Autodesk Inventor part; units mm, degrees
ref_plane "YZ Plane" through (0, 0, 0) normal (1, 0, 0) x (0, 1, 0)
ref_plane "XZ Plane" through (0, 0, 0) normal (0, 1, 0) x (-1, 0, 0)
ref_plane "XY Plane" through (0, 0, 0) normal (0, 0, 1) x (1, 0, 0)
sketch "Sketch1" plane through (0, 0, 0) normal (1, 0, 0) x (0, 1, 0)
  line L0 (10, 0) -> (10, -13)
  line L1 (0, 0) -> (0, -13)
  line L2 (52, -13) -> (52, 55)
  line L3 (52, 55) -> (32, 55)
  line L4 (52, 55) -> (72, 55) construction
  line L5 (32, 55) -> (32, 40)
  line L6 (32, 55) -> (47, 55) construction
  line L7 (32, 40) -> (32, 40)
  line L8 (42, 30) -> (42, -13)
  arc A0 (42, 30) -> (32, 40) centre (32, 30) ccw
  arc A1 (10, -13) -> (42, -13) centre (26, -13) ccw
  arc A2 (0, -13) -> (52, -13) centre (26, -13) ccw
  line L9 (0, 0) -> (10, 0)
  dimension "d2" = 13
  dimension "d7" = 13
  dimension "d12" = 68
  dimension "d14" = 20
  dimension "d16" = 15
  dimension "d19" = 10
  dimension "d20" = 16
  dimension "d21" = 26
  dimension "d22" = 10
extrude "Extrusion1" add sketch "Sketch1" along normal blind 50
sketch "Sketch2" plane through (0, 32, 40) normal (0, -1, 0) x (1, 0, 0)
  circle A0 centre (10, 7.5) radius 2
  line L0 (0, 15) -> (0, 0)
  line L1 (0, 15) -> (50, 15)
  circle A1 centre (40, 7.5) radius 2
  point P0 (0, -40)
  dimension "d25" = 4
  dimension "d26" = 10
  dimension "d27" = 7.5
  dimension "d30" = 30
extrude "Extrusion2" cut sketch "Sketch2" against normal blind 15
properties part number "lid_holder"
Check sheet for the modelled part. Datum: model origin and axes. Units: mm. A direction names the side the tool comes from. Round coordinates to 2 decimals unless told otherwise and drop trailing zeros. Write each loop counter-clockwise with the first axis right and the second up, starting at its lowest first coordinate (ties: lowest second). Pieces come first, ordered by that corner, then holes. Notation, with made-up numbers: (-36.5, 77) -> (-3.5, 77) arc R15 ccw to (-3.5, 96) -> close; hole circle Ø2 at (63.25, 84.5). An arc over 180 degrees is marked (long way). One line per question, with ' | ' between items. Start each with the question number.
1. Set-up check for faces 1 (the face through (25, 10, -6)), 2 (the face through (25, 32, 48)), 3 (the face through (39.566, 39.395, 45.548)): record each of +Z, -Z, +X, -X, +Y, -Y from which the full face is reachable in a straight line by a thin tool's end or side.
2. Sectioned sample at D-D, the plane y = 26. Record the cut outline in (x, z).
3. Release check for a two-part mould opening along X. For faces 4 (the face through (40, 47, 48)), 5 (the face through (50, 43, 5)), 6 (the face through (25, 52, 21)) record: +X half, -X half, draft (parallel to the pull), parting line (faces both ways), or undercut.
4. Sectioned sample at C-C, the plane z = 47.5. Record the cut outline in (x, y).
5. Sectioned sample at B-B, the plane z = -16.5. Record the cut outline in (x, y).
6. Scan lines: line 1 along Y through (x, z) = (43.5, -4.5); line 2 along Z through (x, y) = (10, 40.75); line 3 along Y through (x, z) = (33, 11). Record each from-to range of solid material in increasing order. Write a range as from..to.
7. Depth check by flat-ended pin: pin 1 (3.5 mm diameter, centred on x = 10, z = 47.5, fed in from -Y); pin 2 (4 mm diameter, centred on x = 33.5, z = 15, fed in from -Y); pin 3 (10 mm diameter, centred on x = 14.5, y = 44, fed in from -Z); pin 4 (12 mm diameter, centred on y = 25, z = -21, fed in from -X). Enter the tip coordinate at first touch or a pass-through.
8. Sectioned sample at A-A, the plane x = 40. Record the cut outline in (y, z), then the cut area to 3 significant figures.
Taken from the geometry:
1) face 1: +Z, +X, -X | face 2: +Z, +X, -X, -Y | face 3: -Y
2) outline: (0, -39) -> (50, -39) -> (50, -29) -> (0, -29) -> close
3) face 4: undercut | face 5: +X half | face 6: draft
4) outline: (0, 32) -> (8, 32) -> (8, 47) -> (12, 47) -> (12, 32) -> (38, 32) -> (38, 47) -> (42, 47) -> (42, 32) -> (50, 32) -> (50, 52) -> (0, 52) -> close
5) outline: (0, 0.24) -> (50, 0.24) -> (50, 10.39) -> (0, 10.39) -> close; (0, 41.61) -> (50, 41.61) -> (50, 51.76) -> (0, 51.76) -> close
6) line 1: y = 0..10, 42..52 | line 2: z = -34.41..-19.2, 34.84..45.5, 49.5..55 | line 3: y = 42..52
7) pin 1: stops at y = 47 | pin 2: stops at y = 42 | pin 3: stops at z = -35.52 | pin 4: passes through
8) outline: (0, -13) arc R26 ccw to (52, -13) -> (52, 55) -> (32, 55) -> (32, 49.5) -> (47, 49.5) -> (47, 45.5) -> (32, 45.5) -> (32, 40) arc R10 cw to (42, 30) -> (42, -13) arc R16 cw to (10, -13) -> (10, 0) -> (0, 0) -> close | area: 1,580 mm^2
